from build123d import *

# Parameters (mm, degrees)
SKETCH1_W                 = 570.860988324
SKETCH1_H                 = 315.575
BOSS_EXTRUDE1_DEPTH       = 3.175
SKETCH2_W                 = 3.175
SKETCH2_H                 = 101.6
CUT_EXTRUDE1_DEPTH        = 3.175
SKETCH7_W                 = 50
SKETCH7_H                 = 3.175
CUT_EXTRUDE5_DEPTH        = 3.175
LPATTERN2_COUNT           = 5
LPATTERN2_PITCH           = 91.96
LPATTERN2_COPY_1_SKETCH_W = 3.175
LPATTERN2_COPY_1_SKETCH_H = 101.6
LPATTERN2_COPY_1_DEPTH    = 3.175
LPATTERN2_COPY_2_SKETCH_W = 3.175
LPATTERN2_COPY_2_SKETCH_H = 101.6
LPATTERN2_COPY_2_DEPTH    = 3.175
LPATTERN2_COPY_3_SKETCH_W = 3.175
LPATTERN2_COPY_3_SKETCH_H = 101.6
LPATTERN2_COPY_3_DEPTH    = 3.175
LPATTERN2_COPY_4_SKETCH_W = 3.175
LPATTERN2_COPY_4_SKETCH_H = 101.6
LPATTERN2_COPY_4_DEPTH    = 3.175
SKETCH9_W                 = 34.036
SKETCH9_H                 = 95.25
SKETCH9_R                 = 3.048
SKETCH9_W_2               = 50.8
SKETCH9_H_2               = 33.988
SKETCH9_R_2               = 3
BOSS_EXTRUDE3_DEPTH       = 3.175
SKETCH10_W                = 3.175
SKETCH10_H                = 112.375
CUT_EXTRUDE6_DEPTH        = 373.621475384


with BuildPart() as part:
    # Sketch1 → Boss-Extrude1 (new body)
    with BuildSketch(Plane.XY):
        Rectangle(SKETCH1_W, SKETCH1_H)
    extrude(amount=BOSS_EXTRUDE1_DEPTH)

    # Sketch2 → Cut-Extrude1 (cut)
    with BuildSketch(Plane.XY.offset(3.175)):
        with Locations((-191.887994162, -81.5875)):
            Rectangle(SKETCH2_W, SKETCH2_H)
    cut_extrude1 = extrude(amount=-CUT_EXTRUDE1_DEPTH, mode=Mode.SUBTRACT)

    # Sketch7 → Cut-Extrude5 (cut)
    with BuildSketch(Plane.XY.offset(3.175)):
        with Locations((127.304934912, -156.2)):
            Rectangle(SKETCH7_W, SKETCH7_H)
        with Locations((-55.695065088, -156.2)):
            Rectangle(SKETCH7_W, SKETCH7_H)
    cut_extrude5 = extrude(amount=-CUT_EXTRUDE5_DEPTH, mode=Mode.SUBTRACT)

    # Mirror3: Cut-Extrude1 across plane
    add(cut_extrude1.mirror(Plane.ZX), mode=Mode.SUBTRACT)

    # LPattern2: Cut-Extrude1 ×5
    with Locations(*[(i * LPATTERN2_PITCH, 0, 0) for i in range(1, LPATTERN2_COUNT)]):
        add(cut_extrude1, mode=Mode.SUBTRACT)

    # LPattern2 copy 1 sketch → LPattern2 copy 1 (cut)
    with BuildSketch(Plane(origin=(91.96, 0, 3.175), x_dir=(1, 0, 0), z_dir=(0, 0, 1))):
        with Locations((-191.887994162, 81.5875)):
            Rectangle(LPATTERN2_COPY_1_SKETCH_W, LPATTERN2_COPY_1_SKETCH_H)
    extrude(amount=-LPATTERN2_COPY_1_DEPTH, mode=Mode.SUBTRACT)

    # LPattern2 copy 2 sketch → LPattern2 copy 2 (cut)
    with BuildSketch(Plane(origin=(183.92, 0, 3.175), x_dir=(1, 0, 0), z_dir=(0, 0, 1))):
        with Locations((-191.887994162, 81.5875)):
            Rectangle(LPATTERN2_COPY_2_SKETCH_W, LPATTERN2_COPY_2_SKETCH_H)
    extrude(amount=-LPATTERN2_COPY_2_DEPTH, mode=Mode.SUBTRACT)

    # LPattern2 copy 3 sketch → LPattern2 copy 3 (cut)
    with BuildSketch(Plane(origin=(275.88, 0, 3.175), x_dir=(1, 0, 0), z_dir=(0, 0, 1))):
        with Locations((-191.887994162, 81.5875)):
            Rectangle(LPATTERN2_COPY_3_SKETCH_W, LPATTERN2_COPY_3_SKETCH_H)
    extrude(amount=-LPATTERN2_COPY_3_DEPTH, mode=Mode.SUBTRACT)

    # LPattern2 copy 4 sketch → LPattern2 copy 4 (cut)
    with BuildSketch(Plane(origin=(367.84, 0, 3.175), x_dir=(1, 0, 0), z_dir=(0, 0, 1))):
        with Locations((-191.887994162, 81.5875)):
            Rectangle(LPATTERN2_COPY_4_SKETCH_W, LPATTERN2_COPY_4_SKETCH_H)
    extrude(amount=-LPATTERN2_COPY_4_DEPTH, mode=Mode.SUBTRACT)

    # Sketch9 → Boss-Extrude3 (add)
    # profile 1 of 3: a face of its own
    with BuildSketch(Plane(origin=(0, 0, 0), x_dir=(-1, 0, 0), z_dir=(0, 0, -1))):
        with Locations((-302.448494162, 110.1625)):
            Rectangle(SKETCH9_W, SKETCH9_H)
        with Locations((-304.480494162, 86.35)):
            Circle(SKETCH9_R, mode=Mode.SUBTRACT)
        with Locations((-304.480494162, 133.975)):
            Circle(SKETCH9_R, mode=Mode.SUBTRACT)
    # profile 2 of 3: a face of its own
    with BuildSketch(Plane(origin=(0, 0, 0), x_dir=(-1, 0, 0), z_dir=(0, 0, -1))):
        with Locations((-302.448494162, -110.1625)):
            Rectangle(SKETCH9_W, SKETCH9_H)
        with Locations((-304.480494162, -133.975)):
            Circle(SKETCH9_R, mode=Mode.SUBTRACT)
        with Locations((-304.480494162, -86.35)):
            Circle(SKETCH9_R, mode=Mode.SUBTRACT)
    # profile 3 of 3: a face of its own
    with BuildSketch(Plane(origin=(0, 0, 0), x_dir=(-1, 0, 0), z_dir=(0, 0, -1))):
        with Locations((-260.030494162, -174.7815)):
            Rectangle(SKETCH9_W_2, SKETCH9_H_2)
        with Locations((-260.030494162, -176.8375)):
            Circle(SKETCH9_R_2, mode=Mode.SUBTRACT)
    boss_extrude3 = extrude(amount=-BOSS_EXTRUDE3_DEPTH)

    # Mirror4: Boss-Extrude3 across plane
    add(boss_extrude3.mirror(Plane(origin=(0, 0, 0), x_dir=(0, 0, 1), z_dir=(1, 0, 0))))

    # Mirror5: Cut-Extrude5 across plane
    add(cut_extrude5.mirror(Plane.ZX), mode=Mode.SUBTRACT)

    # Sketch10 → Cut-Extrude6 (cut, through all)
    with BuildSketch(Plane(origin=(0, 0, 0), x_dir=(-1, 0, 0), z_dir=(0, 0, -1))):
        with Locations((-283.842994162, 0)):
            Rectangle(SKETCH10_W, SKETCH10_H)
    cut_extrude6 = extrude(amount=-CUT_EXTRUDE6_DEPTH, mode=Mode.SUBTRACT)

    # Mirror6: Cut-Extrude6 across plane
    add(cut_extrude6.mirror(Plane(origin=(0, 0, 0), x_dir=(0, 0, 1), z_dir=(1, 0, 0))), mode=Mode.SUBTRACT)


solid = part.part
The listing builds one solid part. Answer for the finished solid, in the listing's coordinates (mm). Round coordinates to 2 decimals unless told otherwise and drop trailing zeros. Write each loop counter-clockwise with the first axis right and the second up, starting at its lowest first coordinate (ties: lowest second). Pieces come first, ordered by that corner, then holes. Notation, with made-up numbers: (17, 3.25) - (27, 3.25) arc R14 cw to (27, 29.25) - close; hole circle Ø9 at (9.25, 79). An arc over 180 degrees is marked (long way). Use a Markdown table: item, result. Add a question column.
1. Flat-ended cylindrical pins translate along their axes: P1, Ø1, axis at y = -59.5, z = 1, coming from the -X side; P2, Ø1, axis at x = 181, z = 1, coming from the -Y side; P3, Ø1, axis at y = -169.5, z = 1, coming from the +X side; P4, Ø1.6, axis at y = 62, z = 1.5, coming from the -X side. Find the tip coordinate at first contact, or state that the pin passes through.
2. Consider line 1 (X direction, y = 108, z = 0.9); line 2 (X direction, y = 34, z = 1.85); line 3 (Y direction, x = -149.5, z = 1.45). Determine where each line is inside the solid, lowest interval first.
3. The part is cut by section B-B (z = 2.6). Give the number of separate pieces and of enclosed holes in the cut face, and give its area (3 significant figures).
4. The part is cut by section A-A (y = 114). Write down the section's boundary in (x, z) (1 decimal), and give its area (3 significant figures).
5. The part is cut by section C-C (x = 208.5). Write down the section's boundary in (y, z) (1 decimal).
Reported:
| question | item | result |
|---|---|---|
| 1 | P1 | x = -285.43 |
| 1 | P2 | y = -157.79 |
| 1 | P3 | x = 285.43 |
| 1 | P4 | x = -319.47 |
| 2 | line 1 | -319.47 to -193.48, -190.3 to -101.52, -98.34 to -9.56, -6.38 to 82.4, 85.58 to 174.36, 177.54 to 319.47 |
| 2 | line 2 | -282.26 to -193.48, -190.3 to -101.52, -98.34 to -9.56, -6.38 to 82.4, 85.58 to 174.36, 177.54 to 282.26 |
| 2 | line 3 | -157.79 to 157.79 |
| 3 | separate pieces | 1 |
| 3 | enclosed holes | 20 |
| 3 | area | 192,000 mm^2 |
| 4 | outline | (-319.5, 0) - (-193.5, 0) - (-193.5, 3.2) - (-319.5, 3.2) - close; (-190.3, 0) - (-101.5, 0) - (-101.5, 3.2) - (-190.3, 3.2) - close; (-98.3, 0) - (-9.6, 0) - (-9.6, 3.2) - (-98.3, 3.2) - close; (-6.4, 0) - (82.4, 0) - (82.4, 3.2) - (-6.4, 3.2) - close; (85.6, 0) - (174.4, 0) - (174.4, 3.2) - (85.6, 3.2) - close; (177.5, 0) - (319.5, 0) - (319.5, 3.2) - (177.5, 3.2) - close |
| 4 | area | 1,980 mm^2 |
| 5 | outline | (-157.8, 0) - (157.8, 0) - (157.8, 3.2) - (-157.8, 3.2) - close |
